Verification items for the finished model (mm, model axes). Face numbers are marked on the shaded views. A direction names the side the tool comes from. Give positions to 0.01 mm unless a question says otherwise; leave off trailing zeros. Write each loop counter-clockwise with the first axis right and the second up, starting at its lowest first coordinate (ties: lowest second). Pieces come first, ordered by that corner, then holes. Notation, with made-up numbers: (-15, -34.75) - (44, -34.75) arc R21 cw to (44, -3.75) - close; hole circle Ø6 at (59, 56.25). An arc over 180 degrees is marked (long way). Answer as a JSON object with one key per item and string values. Group by question number.
Item 1: Scan lines: line 1 along Z through (x, y) = (123, 5); line 2 along Y through (x, z) = (97, 127.5); line 3 along X through (y, z) = (2, 125). Record each from-to range of solid material in increasing order. Write a range as [from, to].
Item 2: Go/stop test with flat-tipped pins: pin 1 (10 mm diameter, centred on x = 116.5, z = 108, fed in from -Y); pin 2 (12 mm diameter, centred on y = -5.5, z = 127.5, fed in from +X); pin 3 (4 mm diameter, centred on x = 94, z = 128, fed in from +Y). Record where each tip stops, or that it passes through.
Item 3: Sectioned sample at A-A, the plane y = -1.5. Record the boundary of the cut face in (x, z).
Item 4: Tool access check on the marked faces 1, 2 and 3. Record the directions out of +Z, -Z, +X, -X, +Y, -Y that give a thin tool (end or side, any length) a straight path to the whole face; none if there is none.
Item 5: Sectioned sample at D-D, the plane z = 125.65. Count the separate pieces of the cut face and the enclosed holes in it, and give its area (3 significant figures).
Item 6: Draft check along X on the marked faces 4, 5 and 6. Enter one of: +X half, -X half, draft (parallel to the pull), parting line (faces both ways), or undercut.
Item 7: Sectioned sample at C-C, the plane y = 9. Record the boundary of the cut face in (x, z), and give its area (3 significant figures).
Item 8: Sectioned sample at B-B, the plane z = 108.15. Record the boundary of the cut face in (x, y).
```python
from build123d import *
from build123d.topology import SkipClean

# Parameters (mm, degrees)
ESQUISSE1_R                     = 1.2
BOSS_EXTRU_1_DEPTH              = 20
ENL_V_MAT_EXTRU_1_DEPTH         = 193.532860321
DIAM_TRE_DU_PER_AGE_2_4_2_4_1_D = 2.4
EXTRU_MINCE1_DEPTH              = 10
ENL_V_MAT_EXTRU_2_DEPTH         = 10
CONG_1_R                        = 0.7
CONG_2_R                        = 5


with BuildPart() as part:
    # Esquisse1 → Boss.-Extru.1 (new body)
    with BuildSketch(Plane(origin=(0, 0, 0), x_dir=(1, 0, 0), z_dir=(0, 1, 0))):
        with BuildLine():
            Line((84.027568136, -123.770834875), (92.687822174, -118.770834875))
            Line((92.687822174, -118.770834875), (99.187822174, -130.029165125))
            Line((99.187822174, -130.029165125), (125.168584287, -115.029165125))
            Line((125.168584287, -115.029165125), (118.668584287, -103.770834875))
            Line((118.668584287, -103.770834875), (127.328838325, -98.770834875))
            Line((127.328838325, -98.770834875), (134.227704746, -110.720022031))
            ThreePointArc((134.227704746, -110.720022031), (124.269465579, -121.791214481), (113.401091599, -131.970422535))
            ThreePointArc((113.401091599, -131.970422535), (102.435456053, -134.394500729), (91.418143327, -136.571686604))
            Line((91.418143327, -136.571686604), (84.027568136, -123.770834875))
        make_face()
        with Locations(Location((93.772758664, -125.65, 0), (0, 0, 270))):
            Circle(ESQUISSE1_R, mode=Mode.SUBTRACT)
        with Locations(Location((124.083647797, -108.15, 0), (0, 0, 90))):
            Circle(ESQUISSE1_R, mode=Mode.SUBTRACT)
        with Locations(Location((107.433012702, -129.310254038, 0), (0, 0, 270))):
            Circle(ESQUISSE1_R, mode=Mode.SUBTRACT)
    extrude(amount=BOSS_EXTRU_1_DEPTH)

    # Esquisse2 → Enlèv. mat.-Extru.1 (cut, through all)
    with BuildSketch(Plane(origin=(0, 20, 0), x_dir=(1, 0, 0), z_dir=(0, 1, 0))):
        with BuildLine():
            Line((115.99137931, -127.680264433), (117, -128.790527602))
            ThreePointArc((117, -128.790527602), (125.938380571, -120.064667155), (134.227704746, -110.720022031))
            Line((134.227704746, -110.720022031), (133.426606, -109.332478301))
            ThreePointArc((133.426606, -109.332478301), (125.045964201, -118.82658304), (115.99137931, -127.680264433))
        make_face()
    extrude(amount=-ENL_V_MAT_EXTRU_1_DEPTH, mode=Mode.SUBTRACT)

    # Diamètre du perçage Ø2.4 (2.4)1 (through all)
    with Locations(Plane(origin=(118.194280465, 5, 125.643790397), x_dir=(0.728369799401, 0, -0.685184234583), z_dir=(0.685184234583, 0, 0.728369799401))):
        with Locations((1e-09, 0)):
            Hole(DIAM_TRE_DU_PER_AGE_2_4_2_4_1_D / 2)

    # Esquisse4 → Extru.-Mince1 (add)
    with SkipClean():  # the faces are left unmerged after this step: merging them gives an invalid solid
        with BuildSketch(Plane.XZ):
            with BuildLine():
                Line((84.027568136, 123.770834875), (91.418143327, 136.571686604))
                ThreePointArc((91.418143327, 136.571686604), (102.435456053, 134.394500729), (113.401091599, 131.970422535))
                ThreePointArc((113.401091599, 131.970422535), (115.211517156, 130.392892117), (117, 128.790527602))
                Line((117, 128.790527602), (115.99137931, 127.680264433))
                ThreePointArc((115.99137931, 127.680264433), (118.194363092, 125.643712669), (120.361595403, 123.569156152))
                Line((120.361595403, 123.569156152), (119.314972834, 122.49464175))
                ThreePointArc((119.314972834, 122.49464175), (116.61917678, 125.063854119), (113.868071592, 127.573752285))
                Line((113.868071592, 127.573752285), (114.876730751, 128.6840578))
                ThreePointArc((114.876730751, 128.6840578), (113.79334288, 129.643068138), (112.701949349, 130.592957746))
                ThreePointArc((112.701949349, 130.592957746), (102.466724149, 132.855327369), (92.1861921, 134.901986101))
                Line((92.1861921, 134.901986101), (85.326606241, 123.020834875))
                Line((85.326606241, 123.020834875), (84.027568136, 123.770834875))
            make_face()
        extrude(amount=EXTRU_MINCE1_DEPTH)

    # Esquisse5 → Enlèv. mat.-Extru.2 (cut)
    with SkipClean():  # the faces are left unmerged after this step: merging them gives an invalid solid
        with BuildSketch(Plane(origin=(0, 20, 0), x_dir=(1, 0, 0), z_dir=(0, 1, 0))):
            Polygon((112.17820323, -122.529165125), (91.826606241, -134.279165125), (85.326606241, -123.020834875), (105.67820323, -111.270834875), align=None)
        extrude(amount=-ENL_V_MAT_EXTRU_2_DEPTH, mode=Mode.SUBTRACT)

    # Congé1
    # the kernel refuses this fillet: 0.7 mm, written as the material it adds along each edge
    with BuildSketch(Plane(origin=(125.168584287, 0, 115.029165125), x_dir=(-0.5000000000000003, 0, -0.8660254037844384), z_dir=(0, 1, 0))) as cong_1_piece_1:
        with BuildLine():
            CenterArc((CONG_1_R, CONG_1_R), CONG_1_R, 180, 90)
            Line((0, CONG_1_R), (0, 0))
            Line((0, 0), (CONG_1_R, 0))
        make_face()
    extrude(amount=20)
    with BuildSketch(Plane(origin=(99.187822174, 0, 130.029165125), x_dir=(-0.5000000000000068, 0, -0.8660254037844347), z_dir=(0, 1, 0))) as cong_1_piece_2:
        with BuildLine():
            CenterArc((CONG_1_R, -CONG_1_R), CONG_1_R, 90, 90)
            Line((0, -CONG_1_R), (0, 0))
            Line((0, 0), (CONG_1_R, 0))
        make_face()
    extrude(amount=10)
    with BuildSketch(Plane(origin=(114.876730751, 1.772512212, 128.6840578), x_dir=(-0.7473615518357495, 0, 0.6644175726436354), z_dir=(0, -1, 0))) as cong_1_piece_3:
        with BuildLine():
            CenterArc((0.707566324, 0.699998522), CONG_1_R, 179.384021678, 90.733726194)
            Line((0.007606777, 0.707523972), (0, 0))
            ThreePointArc((0, 0), (0.354502442, -0.000364267), (0.709004885, 0))
        make_face()
    extrude(amount=11.772512212)
    # the kernel refuses this fillet: 0.7 mm, written as the material it takes off along each edge
    with BuildSketch(Plane(origin=(85.326606241, 0, 123.020834875), x_dir=(-0.8660254037844296, 0, 0.5000000000000155), z_dir=(0, -1, 0)), Plane(origin=(85.326606241, 21.75, 123.020834875), x_dir=(-0.8660254037844347, 0, 0.5000000000000068), z_dir=(0, -1, 0)), Plane(origin=(84.027568136, 0, 123.770834875), x_dir=(0.5000000000000003, 0, 0.8660254037844384), z_dir=(0, -1, 0))) as cong_1_2_piece_1:
        with BuildLine():
            CenterArc((CONG_1_R, -CONG_1_R), CONG_1_R, 90, 90)
            Line((0, -CONG_1_R), (0, 0))
            Line((0, 0), (CONG_1_R, 0))
        make_face()
    extrude(amount=11.75, mode=Mode.SUBTRACT)
    with BuildSketch(Plane(origin=(84.027568136, 0, 123.770834875), x_dir=(0.5000000000000003, 0, 0.8660254037844384), z_dir=(0, 1, 0))) as cong_1_2_piece_2:
        with BuildLine():
            CenterArc((CONG_1_R, CONG_1_R), CONG_1_R, 180, 90)
            Line((0, CONG_1_R), (0, 0))
            Line((0, 0), (CONG_1_R, 0))
        make_face()
    extrude(amount=21.75, mode=Mode.SUBTRACT)
    with BuildSketch(Plane(origin=(127.328838325, -1.75, 98.770834875), x_dir=(0.499999999999998, 0, 0.8660254037844398), z_dir=(0, 1, 0)), Plane(origin=(118.668584287, -1.75, 103.770834875), x_dir=(0.8660254037844384, 0, -0.5000000000000003), z_dir=(0, 1, 0))) as cong_1_2_piece_3:
        with BuildLine():
            CenterArc((CONG_1_R, -CONG_1_R), CONG_1_R, 90, 90)
            Line((0, -CONG_1_R), (0, 0))
            Line((0, 0), (CONG_1_R, 0))
        make_face()
    extrude(amount=23.5, mode=Mode.SUBTRACT)
    with BuildSketch(Plane(origin=(133.426606, 21.214506308, 109.332478301), x_dir=(-0.6349000058831564, 0, 0.7725943195038182), z_dir=(0, -1, 0))) as cong_1_2_piece_4:
        with BuildLine():
            CenterArc((0.484816837, 0.699999306), CONG_1_R, 200.587431515, 69.493248031)
            Line((-0.170478849, 0.453853893), (0, 0))
            ThreePointArc((0, 0), (0.242901262, -0.000171018), (0.485802523, 0))
        make_face()
    extrude(amount=22.429012616, mode=Mode.SUBTRACT)
    with BuildSketch(Plane(origin=(92.687822174, -1.75, 118.770834875), x_dir=(-0.8660254037844347, 0, 0.5000000000000068), z_dir=(0, 1, 0))) as cong_1_2_piece_5:
        with BuildLine():
            CenterArc((CONG_1_R, CONG_1_R), CONG_1_R, 180, 90)
            Line((0, CONG_1_R), (0, 0))
            Line((0, 0), (CONG_1_R, 0))
        make_face()
    extrude(amount=13.5, mode=Mode.SUBTRACT)
    with BuildSketch(Plane(origin=(119.314972834, 0, 122.49464175), x_dir=(-0.7177637664774796, 0, 0.6962867049801125), z_dir=(0, -1, 0))) as cong_1_2_piece_6:
        with BuildLine():
            CenterArc((0.698574544, -0.699998546), CONG_1_R, 90.116794283, 89.766411434)
            Line((-0.001424002, -0.698571635), (0, 0))
            ThreePointArc((0, 0), (0.348573817, -0.000355274), (0.697147634, 0))
        make_face()
    extrude(amount=11.746432717, mode=Mode.SUBTRACT)
    with BuildSketch(Plane(origin=(113.868071592, 0, 127.573752285), x_dir=(0.6724137931033691, 0, 0.7401754459885436), z_dir=(0, -1, 0))) as cong_1_2_piece_7:
        with BuildLine():
            CenterArc((0.704715348, -0.7), CONG_1_R, 90, 90.266958587)
            ThreePointArc((0.004722946, -0.703261503), (0.002723014, -0.351628323), (0, 0))
            Line((0, 0), (0.704715348, 0))
        make_face()
    extrude(amount=11.76178837, mode=Mode.SUBTRACT)

    # Congé2
    # the kernel refuses this fillet: 5 mm, written as the material it adds along each edge
    with BuildSketch(Plane(origin=(92.1861921, 8.938383059, 134.901986101), x_dir=(0.9820827402296215, 0, -0.18845023572040911), z_dir=(0, -1, 0))) as cong_2_piece_1:
        with BuildLine():
            CenterArc((3.557422666, -4.999967849), CONG_2_R, 89.794530502, 71.067825025)
            Line((-1.166245932, -3.360774456), (0, 0))
            ThreePointArc((0, 0), (1.787676612, 0.003205414), (3.575353224, 0))
        make_face()
    extrude(amount=18.938383059)
    with BuildSketch(Plane(origin=(112.701949349, 3.163738142, 130.592957746), x_dir=(0.7546589965998223, 0, -0.6561172142620169), z_dir=(0, -1, 0))) as cong_2_piece_2:
        with BuildLine():
            CenterArc((1.247154746, -4.999966362), CONG_2_R, 89.789832754, 28.292116565)
            ThreePointArc((-1.106515, -0.588590304), (-0.553442478, -0.293947404), (0, 0))
            ThreePointArc((0, 0), (0.632747628, 0.001160495), (1.265495257, 0))
        make_face()
    extrude(amount=13.163738142)
    with BuildSketch(Plane(origin=(91.826606241, 20, 134.279165125), x_dir=(0.866025403784453, 0, -0.49999999999997513), z_dir=(0, -1, 0))) as cong_2_piece_3:
        with BuildLine():
            CenterArc((CONG_2_R, -CONG_2_R), CONG_2_R, 90, 90)
            Line((0, -CONG_2_R), (0, 0))
            Line((0, 0), (CONG_2_R, 0))
        make_face()
    extrude(amount=10)
    # the kernel refuses this fillet: 5 mm, written as the material it takes off along each edge
    with BuildSketch(Plane(origin=(113.401091599, -13.143565693, 131.970422535), x_dir=(0.7560908595637044, 1.2400707538838124e-15, -0.6544666623168968), z_dir=(0, 1, 0))) as cong_2_2_piece_1:
        with BuildLine():
            CenterArc((1.239359808, 4.99996736), CONG_2_R, 242.086933336, 28.120093605)
            ThreePointArc((-1.101296945, 0.581672896), (-0.550829587, 0.29049354), (0, 0))
            ThreePointArc((0, 0), (0.628713139, -0.001135866), (1.257426277, 0))
        make_face()
    extrude(amount=36.287131385, mode=Mode.SUBTRACT)
    with BuildSketch(Plane(origin=(91.418143327, -18.917959017, 136.571686604), x_dir=(0.9824849074326925, 0, -0.18634217629665503), z_dir=(0, 1, 0))) as cong_2_2_piece_2:
        with BuildLine():
            CenterArc((3.549347689, 4.999968188), CONG_2_R, 199.260605737, 70.943779261)
            Line((-1.170792196, 3.350641212), (0, 0))
            ThreePointArc((0, 0), (1.783591803, -0.00318121), (3.567183607, 0))
        make_face()
    extrude(amount=47.835918033, mode=Mode.SUBTRACT)
    with BuildSketch(Plane(origin=(95.545706006, -10, 117.120834875), x_dir=(0.5000000000000072, 0, 0.8660254037844346), z_dir=(-0.8660254037844346, 0, 0.5000000000000071))) as cong_2_2_piece_3:
        with BuildLine():
            CenterArc((CONG_2_R, CONG_2_R), CONG_2_R, 180, 90)
            Line((0, CONG_2_R), (0, 0))
            Line((0, 0), (CONG_2_R, 0))
        make_face()
    extrude(amount=25.1, mode=Mode.SUBTRACT)


solid = part.part
```
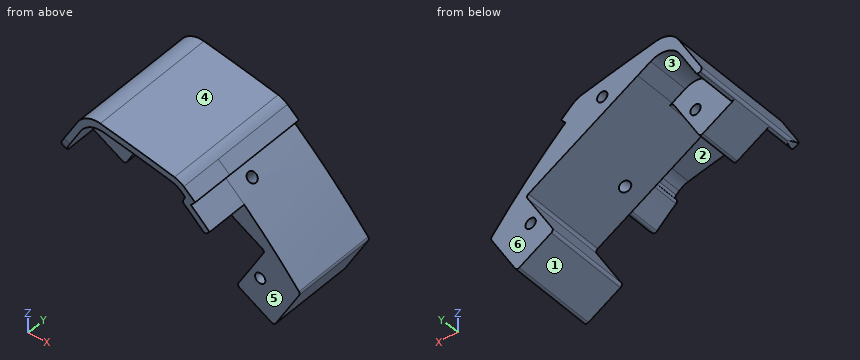
Geometry check:
{
 "1": {"line 1": "[101.27, 107.63], [108.67, 111.27], [116.28, 120.94]", "line 2": "[0, 10]", "line 3": "[84.74, 92.76], [94.78, 96.28], [107.9, 118.87]"},
 "2": {"pin 1": "y = 0", "pin 2": "x = 120.36", "pin 3": "y = 10"},
 "3": {"outline": "(84.38, 124.38) arc R0.7 ccw to (84.63, 123.42) - (84.72, 123.37) arc R0.7 ccw to (85.68, 123.63) - (90.41, 131.82) arc R5 cw to (95.7, 134.23) arc R498.5 cw to (111.48, 130.87) arc R5 cw to (113.66, 129.76) arc R172.5 cw to (114.35, 129.16) arc R0.7 cw to (114.4, 128.16) - (114.34, 128.1) arc R0.7 ccw to (114.39, 127.1) arc R171 cw to (118.81, 122.98) arc R0.7 ccw to (119.8, 123) - (120.36, 123.57) arc R172.5 ccw to (115.99, 127.68) - (117, 128.79) arc R174 ccw to (114.35, 131.15) arc R5 ccw to (112.19, 132.25) arc R500 ccw to (94.92, 135.91) arc R5 ccw to (89.64, 133.5) - close"},
 "4": {"face 1": "-Z, -X, +Y, -Y", "face 2": "-Z, -Y", "face 3": "-Z, +Y"},
 "5": {"separate pieces": "3", "enclosed holes": "0", "area": "372 mm^2"},
 "6": {"face 4": "+X half", "face 5": "undercut", "face 6": "draft"},
 "7": {"outline": "(84.38, 124.38) arc R0.7 ccw to (84.63, 123.42) - (92.08, 119.12) arc R0.7 ccw to (93.04, 119.38) - (98.84, 129.42) arc R0.7 cw to (99.79, 129.68) - (124.56, 115.38) arc R0.7 cw to (124.82, 114.42) - (119.02, 104.38) arc R0.7 ccw to (119.27, 103.42) - (126.72, 99.12) arc R0.7 ccw to (127.68, 99.38) - (133.18, 108.91) arc R0.7 ccw to (133.12, 109.71) arc R172.5 ccw to (115.99, 127.68) - (117, 128.79) arc R174 ccw to (114.35, 131.15) arc R5 ccw to (112.19, 132.25) arc R500 ccw to (94.92, 135.91) arc R5 ccw to (89.64, 133.5) - close; hole circle Ø2.4 at (93.77, 125.65); hole circle Ø2.4 at (107.43, 129.31); hole circle Ø2.4 at (124.08, 108.15)", "area": "471 mm^2"},
 "8": {"outline": "(121.2, 0) - (122.88, 0) - (122.88, 20) - (121.2, 20) - close; (125.28, 0) - (132.74, 0) - (132.74, 20) - (125.28, 20) - close"}
}
